Geometry check sheet. Reference: the model listing, model coordinates, mm. Face numbers are marked on the shaded views. A direction names the side the tool comes from. Give positions to 0.01 mm unless a question says otherwise; leave off trailing zeros. Write each loop counter-clockwise with the first axis right and the second up, starting at its lowest first coordinate (ties: lowest second). Pieces come first, ordered by that corner, then holes. Notation, with made-up numbers: (-22, 42.5) -> (-15, 42.5) arc R7 cw to (-15, 46.5) -> close; hole circle Ø8 at (67.5, 68.5). An arc over 180 degrees is marked (long way). One line per item, written item: value.
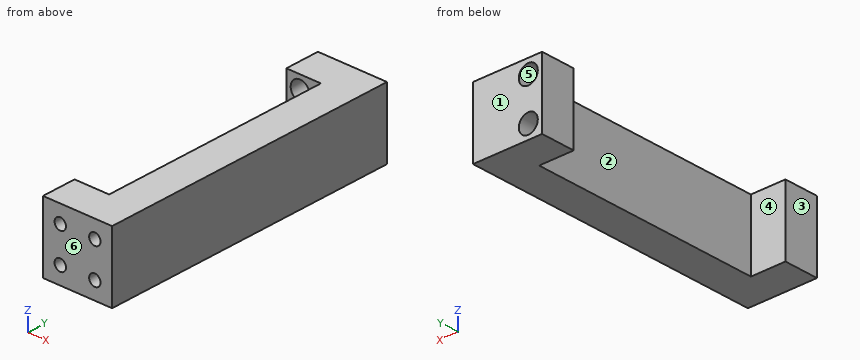
from build123d import *

# Parameters (mm, degrees)
EXTRUDE_1_DEPTH             = 20
HOLE_WIZARD_M4_1_AT_2_COUNT = 2
HOLE_WIZARD_M4_1_AT_2_PITCH = 10
HOLE_WIZARD_M4_1_AT_3_COUNT = 2
HOLE_WIZARD_M4_1_AT_3_PITCH = 10
HOLE_WIZARD_M4_1_AT_4_COUNT = 2
HOLE_WIZARD_M4_1_AT_4_PITCH = 14.142135624
SKETCH_5_W                  = 20
SKETCH_5_H                  = 20
EXTRUDE_2_DEPTH             = 10
SKETCH_6_W                  = 20
SKETCH_6_H                  = 47
CUT_EXTRUDE_2_DEPTH         = 5
SKETCH_7_W                  = 10
SKETCH_7_H                  = 20.15
CUT_EXTRUDE_3_DEPTH         = 21
SKETCH_8_R                  = 2.75
CUT_EXTRUDE_4_DEPTH         = 11


with BuildPart() as part:
    # 草图1 → 凸台-拉伸1 (new body)
    with BuildSketch(Plane.XY):
        Polygon((-20, 30.15), (-15, 30.15), (-15, 77.15), (-20, 77.15), (-20, 87.15), (0, 87.15), (0, 0), (-20, 0), align=None)
    extrude(amount=EXTRUDE_1_DEPTH)

    # 草图3 → M4 螺纹孔1 (revolve, cut)
    with BuildSketch(Plane(origin=(-15, 87.15, 5), x_dir=(0, 0, 1), z_dir=(1, 0, 0))):
        Polygon((0, 0), (0, 6.991420021), (1.65, 6), (1.65, 0), align=None)
    hole_wizard_m4_1 = revolve(axis=Axis((-15, 93.5, 5), (0, -1, 0)), mode=Mode.SUBTRACT)

    # M4 螺纹孔1 at 2: M4 螺纹孔1 ×2
    with Locations(*[(i * HOLE_WIZARD_M4_1_AT_2_PITCH, 0, 0) for i in range(1, HOLE_WIZARD_M4_1_AT_2_COUNT)]):
        add(hole_wizard_m4_1, mode=Mode.SUBTRACT)

    # M4 螺纹孔1 at 3: M4 螺纹孔1 ×2
    with Locations(*[(0, 0, i * HOLE_WIZARD_M4_1_AT_3_PITCH) for i in range(1, HOLE_WIZARD_M4_1_AT_3_COUNT)]):
        add(hole_wizard_m4_1, mode=Mode.SUBTRACT)

    # M4 螺纹孔1 at 4: M4 螺纹孔1 ×2
    with Locations(*[Vector(0.707106781, 0, 0.707106781) * (i * HOLE_WIZARD_M4_1_AT_4_PITCH) for i in range(1, HOLE_WIZARD_M4_1_AT_4_COUNT)]):
        add(hole_wizard_m4_1, mode=Mode.SUBTRACT)

    # 镜向1: M4 螺纹孔1 across plane
    add(hole_wizard_m4_1.mirror(Plane.ZX.offset(43.575)), mode=Mode.SUBTRACT)

    # 镜向1 copy 1 sketch → 镜向1 copy 1 (revolve, cut)
    with BuildSketch(Plane(origin=(-5, 0, 5), x_dir=(0, 0, 1), z_dir=(1, 0, 0))):
        Polygon((0, 0), (0, -6.991420021), (1.65, -6), (1.65, 0), align=None)
    revolve(axis=Axis((-5, -6.35, 5), (0, -1, 0)), mode=Mode.SUBTRACT)

    # 镜向1 copy 2 sketch → 镜向1 copy 2 (revolve, cut)
    with BuildSketch(Plane(origin=(-15, 0, 15), x_dir=(0, 0, 1), z_dir=(1, 0, 0))):
        Polygon((0, 0), (0, -6.991420021), (1.65, -6), (1.65, 0), align=None)
    revolve(axis=Axis((-15, -6.35, 15), (0, -1, 0)), mode=Mode.SUBTRACT)

    # 镜向1 copy 3 sketch → 镜向1 copy 3 (revolve, cut)
    with BuildSketch(Plane(origin=(-5, 0, 15), x_dir=(0, 0, 1), z_dir=(1, 0, 0))):
        Polygon((0, 0), (0, -6.991420021), (1.65, -6), (1.65, 0), align=None)
    revolve(axis=Axis((-5, -6.35, 15), (0, -1, 0)), mode=Mode.SUBTRACT)

    # 草图5 → 凸台-拉伸2 (add)
    with BuildSketch(Plane(origin=(0, 87.15, 0), x_dir=(1, 0, 0), z_dir=(0, 1, 0))):
        with Locations((-10, -10)):
            Rectangle(SKETCH_5_W, SKETCH_5_H)
    extrude(amount=-EXTRUDE_2_DEPTH)

    # 草图6 → 切除-拉伸2 (cut)
    with BuildSketch(Plane.ZY.offset(15)):
        with Locations((10, 53.65)):
            Rectangle(SKETCH_6_W, SKETCH_6_H)
    extrude(amount=-CUT_EXTRUDE_2_DEPTH, mode=Mode.SUBTRACT)

    # 草图7 → 切除-拉伸3 (cut, through all)
    with BuildSketch(Plane.XY.offset(20)):
        with Locations((-15, 20.075)):
            Rectangle(SKETCH_7_W, SKETCH_7_H)
    extrude(amount=-CUT_EXTRUDE_3_DEPTH, mode=Mode.SUBTRACT)

    # 草图8 → 切除-拉伸4 (cut, through all)
    with BuildSketch(Plane.XZ.offset(-77.15)):
        with Locations((-16, 4)):
            Circle(SKETCH_8_R)
        with Locations((-16, 16)):
            Circle(SKETCH_8_R)
    extrude(amount=-CUT_EXTRUDE_4_DEPTH, mode=Mode.SUBTRACT)


solid = part.part
1) Sectioned sample at B-B on y = 73.5. Record the cut outline in (x, z), plus the area to 3 significant figures.
Verdict:
outline: (-10, 0) -> (0, 0) -> (0, 20) -> (-10, 20) -> close
area: 200 mm^2
2) Tool access check on the marked faces 4, 5 and 6. Record the directions out of +Z, -Z, +X, -X, +Y, -Y that give a thin tool (end or side, any length) a straight path to the whole face; none if there is none.
Verdict:
face 4: +Z, -Z, -X
face 5: +Y
face 6: +Z, -Z, +X, -X, -Y
3) Sectioned sample at A-A on x = -12.5. Record the cut outline in (y, z).
Verdict:
outline: (0, 0) -> (10, 0) -> (10, 20) -> (0, 20) -> close; (77.15, 0) -> (87.15, 0) -> (87.15, 20) -> (77.15, 20) -> close
4) Mould release check, pull along Y, two halves, no side actions. Record for the marked faces 1, 2 and 3: released by +Y, released by -Y, zero draft, split by the parting line, or undercut.
Verdict:
face 1: released by +Y
face 2: undercut
face 3: zero draft
5) Scan lines: probe 1 along Z at (x, y) = (-5, 3.15); probe 2 along X at (y, z) = (3.8, 15); probe 3 along Z at (x, y) = (-16, 84.5). Record each from-to range of solid material in increasing order.
Verdict:
probe 1: 0 to 3.35, 6.65 to 13.35, 16.65 to 20
probe 2: -20 to -16.65, -13.35 to -6.65, -3.35 to 0
probe 3: 0 to 1.25, 6.75 to 13.25, 18.75 to 20
6) Depth check by flat-ended pin: pin 1 Ø3.5 at (x, z) = (-16, 16) entering from +Y; pin 2 Ø1.5 at (y, z) = (59, 7.5) entering from -X. Enter the tip coordinate at first touch or a pass-through.
Verdict:
pin 1: y = 10
pin 2: x = -10
